Could you check a few things on this model? Use its own coordinates, in mm. A direction names the side the tool comes from. Coordinates: 2 decimals unless noted, no trailing zeros. Write each loop counter-clockwise with the first axis right and the second up, starting at its lowest first coordinate (ties: lowest second). Pieces come first, ordered by that corner, then holes. Notation, with made-up numbers: (67, 49.25) - (92, 49.25) arc R27 ccw to (92, 78.25) - close; hole circle Ø8 at (26, 37). An arc over 180 degrees is marked (long way). Write item = value, one per line. Start each with the question number.
```python
from build123d import *

# Parameters (mm, degrees)
SKETCH1_W                       = 154
SKETCH1_H                       = 114
SKETCH1_W_2                     = 150
SKETCH1_H_2                     = 110
BOSS_EXTRUDE1_DEPTH             = 2
BOSS_EXTRUDE2_REACH             = 97.823
BOSS_EXTRUDE2_DIRECTION_2_REACH = 97.823
BOSS_EXTRUDE3_DEPTH             = 2
SKETCH4_W                       = 154
SKETCH4_H                       = 31.333333333
SKETCH4_H_2                     = 31.333333334
BOSS_EXTRUDE4_DEPTH             = 2


with BuildPart() as part:
    # Sketch1 → Boss-Extrude1 (new body)
    # profile 1 of 3: a face of its own
    with BuildSketch(Plane(origin=(0, 0, 0), x_dir=(1, 0, 0), z_dir=(0, 1, 0))):
        Rectangle(SKETCH1_W, SKETCH1_H)
        Rectangle(SKETCH1_W_2, SKETCH1_H_2, mode=Mode.SUBTRACT)
    # profile 2 of 3: a face of its own
    with BuildSketch(Plane(origin=(0, 0, 0), x_dir=(1, 0, 0), z_dir=(0, 1, 0))):
        Polygon((-75, 55), (-75, -55), (75, -55), align=None)
    # profile 3 of 3: a face of its own
    with BuildSketch(Plane(origin=(0, 0, 0), x_dir=(1, 0, 0), z_dir=(0, 1, 0))):
        Polygon((75, 55), (75, -55), (-75, 55), align=None)
    extrude(amount=-BOSS_EXTRUDE1_DEPTH)

    # Boss-Extrude2: up to this face of the body (flat: up to its plane)
    boss_extrude2_end = Plane(part.part.faces().sort_by_distance((0, -1, 57))[0])
    # Sketch2 → Boss-Extrude2 (add, up to the picked face)
    with BuildSketch(Plane.XY, mode=Mode.PRIVATE) as boss_extrude2_sk1:
        Polygon((-77, 0), (-77, 13.964466094), (-73.464466094, 17.5), (-73.464466094, 22.5), (-77, 26.035533906), (-77, 38), (-75, 38), (-75, 26.863961031), (-71.464466094, 23.328427125), (-71.464466094, 22.5), (-71.464466094, 17.5), (-71.464466094, 16.671572875), (-75, 13.136038969), (-75, 0), align=None)
    boss_extrude2_tool1 = split(extrude(boss_extrude2_sk1.sketch, amount=BOSS_EXTRUDE2_REACH, mode=Mode.PRIVATE), bisect_by=boss_extrude2_end, keep=Keep.BOTH, mode=Mode.PRIVATE)
    # Sketch2 → Boss-Extrude2 (add, up to the picked face)
    with BuildSketch(Plane.XY, mode=Mode.PRIVATE) as boss_extrude2_sk2:
        Polygon((75, 38), (75, 26.863961031), (71.464466094, 23.328427125), (71.464466094, 22.5), (71.464466094, 17.5), (71.464466094, 16.671572875), (75, 13.136038969), (75, 0), (77, 0), (77, 13.964466094), (73.464466094, 17.5), (73.464466094, 22.5), (77, 26.035533906), (77, 38), align=None)
    boss_extrude2_tool2 = split(extrude(boss_extrude2_sk2.sketch, amount=BOSS_EXTRUDE2_REACH, mode=Mode.PRIVATE), bisect_by=boss_extrude2_end, keep=Keep.BOTH, mode=Mode.PRIVATE)
    add(boss_extrude2_tool1.solids().sort_by(Axis((-76.615989, 6.982233, 0), (0, 0, 1)))[0])
    add(boss_extrude2_tool2.solids().sort_by(Axis((75.384011, 32.431981, 0), (0, 0, 1)))[0])

    # Boss-Extrude2 direction 2: up to this face of the body (flat: up to its plane)
    boss_extrude2_direction_2_end = Plane(part.part.faces().sort_by_distance((0, -1, -57))[0])
    # Sketch2 → Boss-Extrude2 direction 2 (add, up to the picked face)
    with BuildSketch(Plane.XY, mode=Mode.PRIVATE) as boss_extrude2_direction_2_sk1:
        Polygon((-77, 0), (-77, 13.964466094), (-73.464466094, 17.5), (-73.464466094, 22.5), (-77, 26.035533906), (-77, 38), (-75, 38), (-75, 26.863961031), (-71.464466094, 23.328427125), (-71.464466094, 22.5), (-71.464466094, 17.5), (-71.464466094, 16.671572875), (-75, 13.136038969), (-75, 0), align=None)
    boss_extrude2_direction_2_tool1 = split(extrude(boss_extrude2_direction_2_sk1.sketch, amount=-BOSS_EXTRUDE2_DIRECTION_2_REACH, mode=Mode.PRIVATE), bisect_by=boss_extrude2_direction_2_end, keep=Keep.BOTH, mode=Mode.PRIVATE)
    # Sketch2 → Boss-Extrude2 direction 2 (add, up to the picked face)
    with BuildSketch(Plane.XY, mode=Mode.PRIVATE) as boss_extrude2_direction_2_sk2:
        Polygon((75, 38), (75, 26.863961031), (71.464466094, 23.328427125), (71.464466094, 22.5), (71.464466094, 17.5), (71.464466094, 16.671572875), (75, 13.136038969), (75, 0), (77, 0), (77, 13.964466094), (73.464466094, 17.5), (73.464466094, 22.5), (77, 26.035533906), (77, 38), align=None)
    boss_extrude2_direction_2_tool2 = split(extrude(boss_extrude2_direction_2_sk2.sketch, amount=-BOSS_EXTRUDE2_DIRECTION_2_REACH, mode=Mode.PRIVATE), bisect_by=boss_extrude2_direction_2_end, keep=Keep.BOTH, mode=Mode.PRIVATE)
    add(boss_extrude2_direction_2_tool1.solids().sort_by(Axis((-76.615989, 6.982233, 0), (0, 0, -1)))[0])
    add(boss_extrude2_direction_2_tool2.solids().sort_by(Axis((75.384011, 32.431981, 0), (0, 0, -1)))[0])

    # Sketch3 → Boss-Extrude3 (add)
    with BuildSketch(Plane(origin=(0, 0, -57), x_dir=(-1, 0, 0), z_dir=(0, 0, -1))):
        Polygon((-75, 38), (75, 38), (75, 26.863961031), (71.464466094, 23.328427125), (71.464466094, 16.671572875), (75, 13.136038969), (75, 0), (-75, 0), (-75, 13.136038969), (-71.464466094, 16.671572875), (-71.464466094, 23.328427125), (-75, 26.863961031), align=None)
    boss_extrude3 = extrude(amount=-BOSS_EXTRUDE3_DEPTH)

    # Mirror1: Boss-Extrude3 across plane
    add(boss_extrude3.mirror(Plane.XY))

    # Sketch4 → Boss-Extrude4 (add)
    with BuildSketch(Plane.XZ.offset(2)):
        with Locations((0, -41.333333334)):
            Rectangle(SKETCH4_W, SKETCH4_H)
        Rectangle(SKETCH4_W, SKETCH4_H_2)
        with Locations((0, 41.333333334)):
            Rectangle(SKETCH4_W, SKETCH4_H)
    extrude(amount=BOSS_EXTRUDE4_DEPTH)


solid = part.part
```
1) Suppose I cut it at C-C on z = -20. Please give me the cut outline in (x, y), plus the area to 3 significant figures.
2) Suppose I cut it at A-A on x = -14.5. Please give me the cut outline in (y, z), plus the area to 3 significant figures.
3) Thinking about a two-plate mould opening in Z: for faces 1 (the flat face through (-1, 17, -57)), 2 (the flat face through (-1, 19, -55)), 3 (the flat face through (0.4, 38, 55.2)), 4 (the flat face through (-1, 19, 55)), which applies, +Z half, -Z half, draft (parallel to the pull), parting line (faces both ways), or undercut?
4) Suppose I cut it at D-D on z = 30. Please give me the cut outline in (x, y), plus the area to 3 significant figures.
5) For P1, Ø1, axis at x = 14, z = -40, coming from the +Y side; P2, Ø5.5, axis at y = 19, z = 18, coming from the +X side; P3, Ø3.5, axis at y = 21.5, z = 6.5, coming from the -X side, each with a flat end and sliding along its axis, tell me the tip position at first contact or that it passes through.
6) Suppose I cut it at B-B on y = 31. Please give me the cut outline in (x, z), plus the area to 3 significant figures.
7) If I drill on probe 1 along Z at (x, y) = (-20, 8.5); probe 2 along X at (y, z) = (18, 36.5); probe 3 along X at (y, z) = (7.5, 32.5), over which ranges is the centre line in solid material (lowest first)? Write a range as [from, to].
8) Which directions (+Z, -Z, +X, -X, +Y, -Y) give clear straight access to the entire face, cutting with the end or side of a thin tool? Please do faces 5 (the flat face through (73.207, 14.929, 0.77)), 6 (the flat face through (77, 5, -1)), 7 (the flat face through (-1, -2, -21)), 8 (the flat face through (-73.257, 25.121, 0.77)), 9 (the flat face through (-75.207, 24.243, 0.798)).
Reply:
q1.outline = (-77, -2) - (77, -2) - (77, 13.96) - (73.46, 17.5) - (73.46, 22.5) - (77, 26.04) - (77, 38) - (75, 38) - (75, 26.86) - (71.46, 23.33) - (71.46, 16.67) - (75, 13.14) - (75, 0) - (-75, 0) - (-75, 13.14) - (-71.46, 16.67) - (-71.46, 23.33) - (-75, 26.86) - (-75, 38) - (-77, 38) - (-77, 26.04) - (-73.46, 22.5) - (-73.46, 17.5) - (-77, 13.96) - close
q1.area = 472 mm^2
q2.outline = (-4, -57) - (38, -57) - (38, -55) - (0, -55) - (0, 55) - (38, 55) - (38, 57) - (-4, 57) - (-4, 25.67) - (-2, 25.67) - (-2, 15.67) - (-4, 15.67) - (-4, -15.67) - (-2, -15.67) - (-2, -25.67) - (-4, -25.67) - close
q2.area = 568 mm^2
q3.face_1 = -Z half
q3.face_2 = undercut
q3.face_3 = draft
q3.face_4 = undercut
q4.outline = (-77, -4) - (77, -4) - (77, 13.96) - (73.46, 17.5) - (73.46, 22.5) - (77, 26.04) - (77, 38) - (75, 38) - (75, 26.86) - (71.46, 23.33) - (71.46, 16.67) - (75, 13.14) - (75, 0) - (-75, 0) - (-75, 13.14) - (-71.46, 16.67) - (-71.46, 23.33) - (-75, 26.86) - (-75, 38) - (-77, 38) - (-77, 26.04) - (-73.46, 22.5) - (-73.46, 17.5) - (-77, 13.96) - close
q4.area = 780 mm^2
q5.P1 = 0
q5.P2 = 74.71
q5.P3 = -74.21
q6.outline = (-77, -57) - (77, -57) - (77, 57) - (-77, 57) - close; hole (-75, -55) - (75, -55) - (75, 55) - (-75, 55) - close
q6.area = 1,060 mm^2
q7.probe_1 = [-57, -55], [55, 57]
q7.probe_2 = [-73.46, -71.46], [71.46, 73.46]
q7.probe_3 = [-77, -75], [75, 77]
q8.face_5 = none
q8.face_6 = +Z, -Z, +X, +Y, -Y
q8.face_7 = +X, -X, -Y
q8.face_8 = +Y
q8.face_9 = +Z, -Z, -X
